```python
from build123d import *

# Parameters (mm, degrees)
SKETCH1_W           = 70
SKETCH1_H           = 50
BOSS_EXTRUDE1_DEPTH = 5
SKETCH2_W           = 70
SKETCH2_H           = 5
BOSS_EXTRUDE2_DEPTH = 70
SKETCH3_R           = 4.05
CUT_EXTRUDE1_DEPTH  = 10
SKETCH4_R           = 2.5
CUT_EXTRUDE2_DEPTH  = 10
BOSS_EXTRUDE3_DEPTH = 5
BOSS_EXTRUDE4_DEPTH = 5
FILLET1_R           = 4
SKETCH7_R           = 2.1
CUT_EXTRUDE3_DEPTH  = 5


with BuildPart() as part:
    # Sketch1 → Boss-Extrude1 (new body)
    with BuildSketch(Plane(origin=(0, 0, 0), x_dir=(1, 0, 0), z_dir=(0, 1, 0))):
        Rectangle(SKETCH1_W, SKETCH1_H)
    extrude(amount=BOSS_EXTRUDE1_DEPTH)

    # Sketch2 → Boss-Extrude2 (add)
    with BuildSketch(Plane(origin=(0, 5, 0), x_dir=(1, 0, 0), z_dir=(0, 1, 0))):
        with Locations((0, 22.5)):
            Rectangle(SKETCH2_W, SKETCH2_H)
    extrude(amount=BOSS_EXTRUDE2_DEPTH)

    # Sketch3 → Cut-Extrude1 (cut)
    with BuildSketch(Plane(origin=(0, 0, -25), x_dir=(-1, 0, 0), z_dir=(0, 0, -1))):
        with Locations((0, 50)):
            Circle(SKETCH3_R)
    extrude(amount=-CUT_EXTRUDE1_DEPTH, mode=Mode.SUBTRACT)

    # Sketch4 → Cut-Extrude2 (cut)
    with BuildSketch(Plane(origin=(0, 0, -25), x_dir=(-1, 0, 0), z_dir=(0, 0, -1))):
        with Locations((-18.5, 50)):
            Circle(SKETCH4_R)
        with Locations((18.5, 50)):
            Circle(SKETCH4_R)
    extrude(amount=-CUT_EXTRUDE2_DEPTH, mode=Mode.SUBTRACT)

    # Sketch5 → Boss-Extrude3 (add)
    with BuildSketch(Plane(origin=(35, 0, 0), x_dir=(0, 0, -1), z_dir=(1, 0, 0))):
        Polygon((20, 75), (-25, 5), (20, 5), align=None)
    extrude(amount=-BOSS_EXTRUDE3_DEPTH)

    # Sketch6 → Boss-Extrude4 (add)
    with BuildSketch(Plane.ZY.offset(35)):
        Polygon((-20, 75), (25, 5), (-20, 5), align=None)
    extrude(amount=-BOSS_EXTRUDE4_DEPTH)

    # Fillet1
    fillet1_edges = [part.edges().sort_by_distance(p)[0] for p in [
        (30, 40, -20),
        (30, 5, 2.5),
        (0, 5, -20),
        (-30, 40, -20),
        (-30, 5, 2.5),
    ]]
    fillet(fillet1_edges, radius=FILLET1_R)

    # Sketch7 → Cut-Extrude3 (cut)
    with BuildSketch(Plane(origin=(0, 5, 0), x_dir=(1, 0, 0), z_dir=(0, 1, 0))):
        with Locations(Location((-15, 5, 0), (0, 0, 270))):
            Circle(SKETCH7_R)
        with Locations(Location((15, 5, 0), (0, 0, 270))):
            Circle(SKETCH7_R)
        with Locations(Location((15, -15, 0), (0, 0, 270))):
            Circle(SKETCH7_R)
        with Locations(Location((-15, -15, 0), (0, 0, 270))):
            Circle(SKETCH7_R)
    extrude(amount=-CUT_EXTRUDE3_DEPTH, mode=Mode.SUBTRACT)


solid = part.part
```
Design review of the part built by this model. Coordinates are the model's own, in mm. A direction names the side the tool comes from. Coordinates: 2 decimals unless noted, no trailing zeros. Loops run counter-clockwise (first coordinate to the right, second up) from the corner with the lowest first, then second, coordinate; pieces in that order, holes last. Notation, with made-up numbers: (84, -1.75) -> (117, -1.75) arc R14 ccw to (117, 8.25) -> close; hole circle Ø4 at (-28.75, 20). An arc over 180 degrees is marked (long way). Answer as a JSON object with one key per item and string values.
Q1. Tool access review of faces 5 (the cylindrical face through (28.797, 6.141, 4.213)), 6 (the flat face through (0, 75, -23)): name each direction out of +Z, -Z, +X, -X, +Y, -Y from which nothing blocks a thin tool from reaching the whole face with its end or side.
Answer block:
{"face 5": "+Z, +Y", "face 6": "+Z, -Z, +X, -X, +Y"}
Q2. Take a section at A-A on x = -15. Give the boundary of the cut face in (y, z).
Answer block:
{"outline": "(0, -25) -> (75, -25) -> (75, -20) -> (9, -20) arc R4 cw to (5, -16) -> (5, -7.1) -> (0, -7.1) -> close; (0, -2.9) -> (5, -2.9) -> (5, 12.9) -> (0, 12.9) -> close; (0, 17.1) -> (5, 17.1) -> (5, 25) -> (0, 25) -> close"}
Q3. Take a section at B-B on z = -5. Give the boundary of the cut face in (x, y).
Answer block:
{"outline": "(-35, 0) -> (-17.1, 0) -> (-17.1, 5) -> (-26, 5) arc R4 cw to (-30, 9) -> (-30, 51.67) -> (-35, 51.67) -> close; (-12.9, 0) -> (12.9, 0) -> (12.9, 5) -> (-12.9, 5) -> close; (17.1, 0) -> (35, 0) -> (35, 51.67) -> (30, 51.67) -> (30, 9) arc R4 cw to (26, 5) -> (17.1, 5) -> close"}
Q4. The part is to be moulded in two halves that separate along Y. For faces 1 (the flat face through (0, 5, 4)), 2 (the flat face through (0, 42, -20)), 3 (the cylindrical face through (0.527, 54.016, -22.535)), 4 (the flat face through (0, 0, 0)), say which applies: +Y half, -Y half, draft (parallel to the pull), parting line (faces both ways), or undercut.
Answer block:
{"face 1": "+Y half", "face 2": "draft", "face 3": "undercut", "face 4": "-Y half"}
Q5. To check wall thickness, follow L1, parallel to X at y = 3.8, z = 15; L2, parallel to Y at x = -18.5, z = -20.95; L3, parallel to X at y = 41, z = -16. State the ranges of each line that lie inside material, in increasing order.
Answer block:
{"L1": "x = -35 to -17.1, -12.9 to 12.9, 17.1 to 35", "L2": "y = 0 to 47.5, 52.5 to 75", "L3": "x = -35 to -30, 30 to 35"}
Q6. Take a section at C-C on x = 0. Give the boundary of the cut face in (y, z), plus the area to 3 significant figures.
Answer block:
{"outline": "(0, -25) -> (45.95, -25) -> (45.95, -20) -> (9, -20) arc R4 cw to (5, -16) -> (5, 25) -> (0, 25) -> close; (54.05, -25) -> (75, -25) -> (75, -20) -> (54.05, -20) -> close", "area": "563 mm^2"}
Q7. Clearance check with flat-ended pins moving along their axes: pin 1 Ø8 at (x, y) = (-18.5, 50) entering from +Z; pin 2 Ø12 at (x, z) = (19, 5) entering from +Y; pin 3 Ø3.5 at (x, z) = (-15, -5) entering from -Y. State where each tip first meets the part, or that it passes through.
Answer block:
{"pin 1": "stops at z = -20", "pin 2": "stops at y = 5", "pin 3": "passes through"}
Q8. Take a section at D-D on y = 50. Give the boundary of the cut face in (x, z), plus the area to 3 significant figures.
Answer block:
{"outline": "(-35, -25) -> (-21, -25) -> (-21, -20) -> (-26, -20) arc R4 cw to (-30, -16) -> (-30, -3.93) -> (-35, -3.93) -> close; (-16, -25) -> (-4.05, -25) -> (-4.05, -20) -> (-16, -20) -> close; (4.05, -25) -> (16, -25) -> (16, -20) -> (4.05, -20) -> close; (21, -25) -> (35, -25) -> (35, -3.93) -> (30, -3.93) -> (30, -16) arc R4 cw to (26, -20) -> (21, -20) -> close", "area": "427 mm^2"}
